Verification items for the finished model (mm, model axes). Give positions to 0.01 mm unless a question says otherwise; leave off trailing zeros. Write each loop counter-clockwise with the first axis right and the second up, starting at its lowest first coordinate (ties: lowest second). Pieces come first, ordered by that corner, then holes. Notation, with made-up numbers: M 49,45.5 L 97,45.5 A30 cw 97,74.5 Z; hole C 24.5,69.5 d2. An arc over 180 degrees is marked long. Answer as a JSON object with one key per item and string values.
```python
from build123d import *

# Parameters (mm, degrees)
CYLINDER_R       = 0.51
CYLINDER_DEPTH   = 3.2
ARRAY001_X_COUNT = 5
ARRAY001_X_PITCH = 2.54
ARRAY001_Y_COUNT = 5
ARRAY001_Y_PITCH = 2.54
BOX002_W         = 10.16
BOX002_H         = 1
BOX002_DEPTH     = 0.035
ARRAY002_Y_COUNT = 2
ARRAY002_Y_PITCH = 9.16
BOX001_W         = 10.16
BOX001_H         = 2
BOX001_DEPTH     = 0.035
ARRAY_Y_COUNT    = 3
ARRAY_Y_PITCH    = 2.54
BOX_W            = 10.16
BOX_H            = 10.16
BOX_DEPTH        = 1.6


with BuildPart() as arraycylinders:
    # Cylinder → Cylinder (new body)
    with BuildSketch(Plane.XY.offset(-0.8)):
        Circle(CYLINDER_R)
    extrude(amount=CYLINDER_DEPTH)

    # Array001 X: ArrayCylinders ×5


with BuildPart() as arraycylinders_1:
    add(arraycylinders.part)
    with Locations(*[(i * ARRAY001_X_PITCH, 0, 0) for i in range(1, ARRAY001_X_COUNT)]):
        add(arraycylinders.part)

    # Array001 Y: ArrayCylinders ×5


with BuildPart() as arraycylinders_2:
    add(arraycylinders_1.part)
    with Locations(*[(0, i * ARRAY001_Y_PITCH, 0) for i in range(1, ARRAY001_Y_COUNT)]):
        add(arraycylinders_1.part)


with BuildPart() as array002:
    # Box002 → Box002 (new body)
    with BuildSketch(Plane.XY.offset(-0.035)):
        with Locations((5.08, 0.5)):
            Rectangle(BOX002_W, BOX002_H)
    extrude(amount=BOX002_DEPTH)

    # Array002 Y: Array002 ×2


with BuildPart() as array002_1:
    add(array002.part)
    with Locations(*[(0, i * ARRAY002_Y_PITCH, 0) for i in range(1, ARRAY002_Y_COUNT)]):
        add(array002.part)


with BuildPart() as fusion:
    # Box001 → Box001 (new body)
    with BuildSketch(Plane(origin=(0, 1.54, -0.035), x_dir=(1, 0, 0), z_dir=(0, 0, 1))):
        with Locations((5.08, 1)):
            Rectangle(BOX001_W, BOX001_H)
    extrude(amount=BOX001_DEPTH)

    # Array Y: Fusion ×3


with BuildPart() as fusion_1:
    add(fusion.part)
    with Locations(*[(0, i * ARRAY_Y_PITCH, 0) for i in range(1, ARRAY_Y_COUNT)]):
        add(fusion.part)

    # Fusion: union Array002
    add(array002_1.part)


with BuildPart() as cut:
    # Box → Box (new body)
    with BuildSketch(Plane.XY):
        with Locations((5.08, 5.08)):
            Rectangle(BOX_W, BOX_H)
    extrude(amount=BOX_DEPTH)

    # Fusion001: union Fusion
    add(fusion_1.part)

    # Cut: cut ArrayCylinders
    add(arraycylinders_2.part, mode=Mode.SUBTRACT)


solid = cut.part
```
1) Section check B-B on y = 7.62. Record the boundary of the cut face in (x, z) (3 decimals), and give its area (3 significant figures).
Completed:
{"outline": "M 0.51,-0.035 L 2.03,-0.035 L 2.03,1.6 L 0.51,1.6 Z; M 3.05,-0.035 L 4.57,-0.035 L 4.57,1.6 L 3.05,1.6 Z; M 5.59,-0.035 L 7.11,-0.035 L 7.11,1.6 L 5.59,1.6 Z; M 8.13,-0.035 L 9.65,-0.035 L 9.65,1.6 L 8.13,1.6 Z", "area": "9.94 mm2"}
2) Release check for a two-part mould opening along Y. For faces 1 (the face through (5, 9.4, -0.035)), 2 (the face through (5.09, 0.51, 0.77)), 3 (the face through (5.014, 5.586, 0.771)), 4 (the face through (7.61, 9.65, 0.77)) record: pulls with the +Y half, pulls with the -Y half, needs draft (parallel to the pull), parting line crosses it, or undercut.
Completed:
{"face 1": "needs draft", "face 2": "pulls with the -Y half", "face 3": "undercut", "face 4": "pulls with the +Y half"}
3) Thickness scan on L1, parallel to X at y = 5.08, z = 1.05; L2, parallel to Z at x = 5.5, y = 9. Record the ranges inside material, lowest first.
Completed:
{"L1": "x = 0.51 to 2.03, 3.05 to 4.57, 5.59 to 7.11, 8.13 to 9.65", "L2": "z = 0 to 1.6"}
4) Section check A-A on x = 5.08. Count the separate pieces of the cut face and the enclosed holes in it, and give its area (3 significant figures).
Completed:
{"separate pieces": "4", "enclosed holes": "0", "area": "9.87 mm2"}
5) Go/stop test with a flat-tipped pin: pin 1 (0.6 mm diameter, centred on x = 5.08, y = 7.62, fed in from -Z). Record where the tip stops, or that it passes through.
Completed:
{"pin 1": "passes through"}
